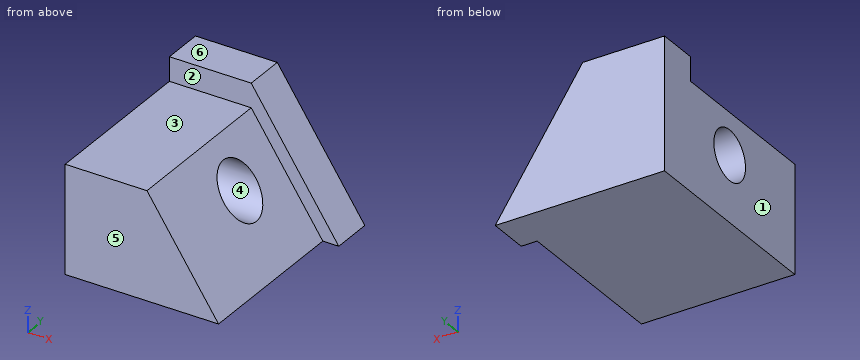
from build123d import *

# Parameters (mm, degrees)
F1_DEPTH = 63.5
F2_R     = 7.718493
F3_DEPTH = 52.580988
F5_DEPTH = 50.8


with BuildPart() as f1:
    # F0 (on Front) → F1 (new body)
    with BuildSketch(Plane.XZ):
        Polygon((-52.579988, 0), (0, 0), (-27.184211, 40.955156), (-52.579988, 40.955156), align=None)
    extrude(amount=F1_DEPTH)

    # F2 (on Right) → F3 (cut, through all)
    with BuildSketch(Plane.YZ):
        with Locations((-31.75, 20.477578)):
            Circle(F2_R)
    extrude(amount=-F3_DEPTH, mode=Mode.SUBTRACT)

    # F4 (on face) → F5 (cut)
    with BuildSketch(Plane.XZ.offset(63.5)):
        Polygon((-52.579988, 40.955156), (-52.579988, 33.481799), (-27.184211, 33.481799), (-4.960482, 0), (0, 0), (-27.184211, 40.955156), align=None)
    extrude(amount=-F5_DEPTH, mode=Mode.SUBTRACT)


solid = f1.part
Check sheet for the modelled part. Datum: model origin and axes. Units: mm. Face numbers are marked on the shaded views. A direction names the side the tool comes from. Give positions to 0.01 mm unless a question says otherwise; leave off trailing zeros. Order: outer loops, then holes, each group sorted by start corner. A loop starts at its lowest first (then second) coordinate and runs counter-clockwise, first axis right, second up. Notation, with made-up numbers: (19, 87.5) - (69, 87.5) arc R36 cw to (69, 125.5) - close; hole circle Ø5 at (29.5, 12). An arc over 180 degrees is marked (long way). Answer as CSV lines item,"result".
1. Section check B-B (y = -31.75). Record the boundary of the cut face in (x, z), then the cut area to 3 significant figures.
Result sheet:
outline,"(-52.58, 0) - (-4.96, 0) - (-13.43, 12.76) - (-52.58, 12.76) - close; (-52.58, 28.2) - (-23.68, 28.2) - (-27.18, 33.48) - (-52.58, 33.48) - close"
area,"697 mm²"
2. Section check D-D (y = -11). Record the boundary of the cut face in (x, z), then the cut area to 3 significant figures.
Result sheet:
outline,"(-52.58, 0) - (0, 0) - (-27.18, 40.96) - (-52.58, 40.96) - close"
area,"1,600 mm²"
3. Section check A-A (z = 19.5). Record the boundary of the cut face in (x, y).
Result sheet:
outline,"(-52.58, -63.5) - (-17.9, -63.5) - (-17.9, -39.41) - (-52.58, -39.41) - close; (-52.58, -24.09) - (-17.9, -24.09) - (-17.9, -12.7) - (-12.94, -12.7) - (-12.94, 0) - (-52.58, 0) - close"
4. Scan lines: probe 1 along Z at (x, y) = (-27.5, -31.75); probe 2 along Z at (x, y) = (-27.5, -43.5); probe 3 along Y at (x, z) = (-43.5, 16). Record each from-to range of solid material in increasing order. Write a range as from..to.
Result sheet:
probe 1,"0..12.76, 28.2..33.48"
probe 2,"0..33.48"
probe 3,"-63.5..-38.04, -25.46..0"
5. Go/stop test with flat-tipped pins: P1, Ø5, axis at y = -39.5, z = 27, coming from the +X side; P2, Ø20.5, axis at x = -35, y = -43.5, coming from the +Z side; P3, Ø5, axis at y = -26, z = 26.5, coming from the +X side. Record where each tip stops, or that it passes through.
Result sheet:
P1,"x = -21.22"
P2,"z = 33.48"
P3,"x = -21.03"
6. Mould release check, pull along Y, two halves, no side actions. Record for the marked faces 4, 5 and 6: released by +Y, released by -Y, zero draft, split by the parting line, or undercut.
Result sheet:
face 4,"undercut"
face 5,"released by -Y"
face 6,"zero draft"
7. Section check C-C (x = -38.5). Record the boundary of the cut face in (y, z).
Result sheet:
outline,"(-63.5, 0) - (0, 0) - (0, 40.96) - (-12.7, 40.96) - (-12.7, 33.48) - (-63.5, 33.48) - close; hole circle Ø15.44 at (-31.75, 20.48)"
8. Tool access check on the marked faces 1, 2 and 3. Record the directions out of +Z, -Z, +X, -X, +Y, -Y that give a thin tool (end or side, any length) a straight path to the whole face; none if there is none.
Result sheet:
face 1,"+Z, -Z, -X, +Y, -Y"
face 2,"+Z, +X, -Y"
face 3,"+Z, +X, -X, -Y"
